Build history of the part. All positions in model axes, mm. Give positions to 0.01 mm unless a question says otherwise; leave off trailing zeros. Write each loop counter-clockwise with the first axis right and the second up, starting at its lowest first coordinate (ties: lowest second). Pieces come first, ordered by that corner, then holes. Notation, with made-up numbers: (81, 7) -> (88, 7) arc R28 ccw to (88, 38) -> close; hole circle Ø5 at (-5, -1.5). An arc over 180 degrees is marked (long way). Put each result on its own line as item: value. Start each with the question number.
Item 1: Flat gauge pins, fed straight in: pin 1 Ø1 at (x, z) = (-97, 20.5) entering from +Y; pin 2 Ø15 at (x, y) = (-25, 25) entering from +Z; pin 3 Ø4 at (y, z) = (40, 19.5) entering from +X. Where does each tip first touch, or does it go through?
Item 2: Two-plate mould, pull along X, no slides. Class faces 1 (the cylindrical face through (-587.488, 25.55, 12.325)), 2 (the cylindrical face through (-2, 46, 13)), 3 (the flat face through (-304, 25, 0)): pulls with the +X half, pulls with the -X half, needs draft (parallel to the pull), parting line crosses it, or undercut.
Item 3: Slice it at A-A, the plane y = 25. List the corners of the cut face in (x, z).
Item 4: Drill centre lines: line 1 along Y through (x, z) = (-575, 14); line 2 along X through (y, z) = (25.5, 20.5); line 3 along X through (y, z) = (23, 21). Where is each one in solid material? Low to high.
Item 5: Slice it at B-B, the plane x = -575. List the corners of the cut face in (y, z), plus the area to 3 significant figures.
Item 6: Slice it at C-C, the plane x = -302. List the corners of the cut face in (y, z), plus the area to 3 significant figures.
```python
from build123d import *

# Parameters (mm, degrees)
SKETCH1_W           = 600
SKETCH1_H           = 50
SKETCH1_R           = 12.5
BOSS_EXTRUDE2_DEPTH = 25
FILLET2_R           = 10


with BuildPart() as part:
    # Sketch1 → Boss-Extrude2 (new body)
    with BuildSketch(Plane.XY):
        with Locations((-300, 25)):
            Rectangle(SKETCH1_W, SKETCH1_H)
        with Locations((-575, 25)):
            Circle(SKETCH1_R, mode=Mode.SUBTRACT)
        with Locations((-25, 25)):
            Circle(SKETCH1_R, mode=Mode.SUBTRACT)
    extrude(amount=BOSS_EXTRUDE2_DEPTH)

    # Fillet2
    fillet2_edges = [part.edges().sort_by_distance(p)[0] for p in [
        (-300, 0, 25),
        (-300, 0, 0),
        (-300, 50, 0),
        (-300, 50, 25),
        (0, 0, 12.5),
        (-600, 0, 12.5),
        (-600, 50, 12.5),
        (0, 50, 12.5),
    ]]
    fillet(fillet2_edges, radius=FILLET2_R)


solid = part.part
```
Values follow:
1. pin 1: y = 48.66
1. pin 2: through
1. pin 3: x = 0
2. face 1: undercut
2. face 2: pulls with the +X half
2. face 3: needs draft
3. outline: (-600, 0) -> (-587.5, 0) -> (-587.5, 25) -> (-600, 25) -> close; (-562.5, 0) -> (-37.5, 0) -> (-37.5, 25) -> (-562.5, 25) -> close; (-12.5, 0) -> (0, 0) -> (0, 25) -> (-12.5, 25) -> close
4. line 1: 0 to 12.5, 37.5 to 50
4. line 2: -600 to -587.49, -562.51 to -37.49, -12.51 to 0
4. line 3: -600 to -587.34, -562.66 to -37.34, -12.66 to 0
5. outline: (0, 10) arc R10 ccw to (10, 0) -> (12.5, 0) -> (12.5, 25) -> (10, 25) arc R10 ccw to (0, 15) -> close; (37.5, 0) -> (40, 0) arc R10 ccw to (50, 10) -> (50, 15) arc R10 ccw to (40, 25) -> (37.5, 25) -> close
5. area: 539 mm2
6. outline: (0, 10) arc R10 ccw to (10, 0) -> (40, 0) arc R10 ccw to (50, 10) -> (50, 15) arc R10 ccw to (40, 25) -> (10, 25) arc R10 ccw to (0, 15) -> close
6. area: 1,160 mm2
